from build123d import *
from OCP.BRepFilletAPI import BRepFilletAPI_MakeChamfer

# Parameters (mm, degrees)
SKETCH1_W                = 11.43
SKETCH1_H                = 6.096
BASE_EXTRUDE_DEPTH       = 3.81
CHAMFER1_SIZE            = 2.159
CHAMFER1_SIZE2           = 0.380689951
CHAMFER2_SIZE            = 1.27
CHAMFER2_SIZE2           = 0.111110603
CUT_EXTRUDE1_DEPTH       = 0.254
BOSS_EXTRUDE_THIN1_DEPTH = 0.635
CUT_EXTRUDE2_DEPTH       = 0.254
CUT_EXTRUDE3_DEPTH       = 0.254
LPATTERN1_COUNT          = 4
LPATTERN1_PITCH          = 2.54
MIRROR1_COPY_1_DEPTH     = 0.635
MIRROR1_COPY_2_DEPTH     = 0.635
MIRROR1_COPY_3_DEPTH     = 0.635
MIRROR1_COPY_4_DEPTH     = 0.254
MIRROR1_COPY_5_DEPTH     = 0.254
MIRROR1_COPY_6_DEPTH     = 0.254
MIRROR1_COPY_7_DEPTH     = 0.254
MIRROR1_COPY_8_DEPTH     = 0.254
MIRROR1_COPY_9_DEPTH     = 0.254


with BuildPart() as part:
    # Sketch1 → Base-Extrude (new body)
    with BuildSketch(Plane(origin=(0, 0.381, 0), x_dir=(0, 0, -1), z_dir=(0, 1, 0))):
        with Locations((-3.81, -3.81)):
            Rectangle(SKETCH1_W, SKETCH1_H)
    extrude(amount=BASE_EXTRUDE_DEPTH)

    # Chamfer1: one chamfer whose edges measure the first distance from different faces: ONE call of the kernel's chamfer builder (chamfer() names one face for all edges)
    chamfer1_edges_1 = [part.edges().sort_by_distance(p)[0] for p in [
        (3.81, 4.191, 9.525),
    ]]
    chamfer1_side_1 = [part.faces().sort_by_distance(p)[0] for p in [
        (3.81, 2.286, 9.525),
    ]]
    chamfer1_edges_2 = [part.edges().sort_by_distance(p)[0] for p in [
        (6.858, 4.191, 3.81),
    ]]
    chamfer1_side_2 = [part.faces().sort_by_distance(p)[0] for p in [
        (6.858, 2.286, 3.81),
    ]]
    chamfer1_edges_3 = [part.edges().sort_by_distance(p)[0] for p in [
        (3.81, 4.191, -1.905),
    ]]
    chamfer1_side_3 = [part.faces().sort_by_distance(p)[0] for p in [
        (3.81, 2.286, -1.905),
    ]]
    chamfer1_edges_4 = [part.edges().sort_by_distance(p)[0] for p in [
        (0.762, 4.191, 3.81),
    ]]
    chamfer1_side_4 = [part.faces().sort_by_distance(p)[0] for p in [
        (0.762, 2.286, 3.81),
    ]]
    chamfer1 = BRepFilletAPI_MakeChamfer(part.part.solid().wrapped)
    for e in chamfer1_edges_1:
        chamfer1.Add(CHAMFER1_SIZE, CHAMFER1_SIZE2, e.wrapped, chamfer1_side_1[0].wrapped)  # the first distance lies on this face
    for e in chamfer1_edges_2:
        chamfer1.Add(CHAMFER1_SIZE, CHAMFER1_SIZE2, e.wrapped, chamfer1_side_2[0].wrapped)  # the first distance lies on this face
    for e in chamfer1_edges_3:
        chamfer1.Add(CHAMFER1_SIZE, CHAMFER1_SIZE2, e.wrapped, chamfer1_side_3[0].wrapped)  # the first distance lies on this face
    for e in chamfer1_edges_4:
        chamfer1.Add(CHAMFER1_SIZE, CHAMFER1_SIZE2, e.wrapped, chamfer1_side_4[0].wrapped)  # the first distance lies on this face
    add(Compound.cast(chamfer1.Shape()), mode=Mode.REPLACE)

    # Chamfer2: one chamfer whose edges measure the first distance from different faces: ONE call of the kernel's chamfer builder (chamfer() names one face for all edges)
    chamfer2_edges_1 = [part.edges().sort_by_distance(p)[0] for p in [
        (6.858, 0.381, 3.81),
    ]]
    chamfer2_side_1 = [part.faces().sort_by_distance(p)[0] for p in [
        (6.858, 1.2065, 3.81),
    ]]
    chamfer2_edges_2 = [part.edges().sort_by_distance(p)[0] for p in [
        (3.81, 0.381, 9.525),
    ]]
    chamfer2_side_2 = [part.faces().sort_by_distance(p)[0] for p in [
        (3.81, 1.2065, 9.525),
    ]]
    chamfer2_edges_3 = [part.edges().sort_by_distance(p)[0] for p in [
        (0.762, 0.381, 3.81),
    ]]
    chamfer2_side_3 = [part.faces().sort_by_distance(p)[0] for p in [
        (0.762, 1.2065, 3.81),
    ]]
    chamfer2_edges_4 = [part.edges().sort_by_distance(p)[0] for p in [
        (3.81, 0.381, -1.905),
    ]]
    chamfer2_side_4 = [part.faces().sort_by_distance(p)[0] for p in [
        (3.81, 1.2065, -1.905),
    ]]
    chamfer2 = BRepFilletAPI_MakeChamfer(part.part.solid().wrapped)
    for e in chamfer2_edges_1:
        chamfer2.Add(CHAMFER2_SIZE, CHAMFER2_SIZE2, e.wrapped, chamfer2_side_1[0].wrapped)  # the first distance lies on this face
    for e in chamfer2_edges_2:
        chamfer2.Add(CHAMFER2_SIZE, CHAMFER2_SIZE2, e.wrapped, chamfer2_side_2[0].wrapped)  # the first distance lies on this face
    for e in chamfer2_edges_3:
        chamfer2.Add(CHAMFER2_SIZE, CHAMFER2_SIZE2, e.wrapped, chamfer2_side_3[0].wrapped)  # the first distance lies on this face
    for e in chamfer2_edges_4:
        chamfer2.Add(CHAMFER2_SIZE, CHAMFER2_SIZE2, e.wrapped, chamfer2_side_4[0].wrapped)  # the first distance lies on this face
    add(Compound.cast(chamfer2.Shape()), mode=Mode.REPLACE)

    # Sketch2 → Cut-Extrude1 (cut)
    with BuildSketch(Plane(origin=(0, 4.191, 0), x_dir=(-1, 0, 0), z_dir=(0, 1, 0))):
        with BuildLine():
            Line((-2.794, -2.791910465), (-4.826, -2.791910465))
            Line((-4.826, -2.791910465), (-4.826, -0.508310049))
            ThreePointArc((-4.826, -0.508310049), (-3.81, 0.507689951), (-2.794, -0.508310049))
            Line((-2.794, -0.508310049), (-2.794, -2.791910465))
        make_face()
    extrude(amount=-CUT_EXTRUDE1_DEPTH, mode=Mode.SUBTRACT)

    # Sketch3 → Boss-Extrude-Thin1 (add, symmetric)
    with BuildSketch(Plane(origin=(9.017, 0, 0), x_dir=(-1, 0, 0), z_dir=(0, 0, -1))):
        with BuildLine():
            Line((6.913298214, 1.778), (8.509, 1.778))
            ThreePointArc((8.509, 1.778), (8.778407684, 1.666407684), (8.89, 1.397))
            Line((8.89, 1.397), (8.89, -2.667))
            Line((8.89, -2.667), (9.144, -2.667))
            Line((9.144, -2.667), (9.144, 1.397))
            ThreePointArc((9.144, 1.397), (8.958012806, 1.846012806), (8.509, 2.032))
            Line((8.509, 2.032), (6.913298214, 2.032))
            Line((6.913298214, 2.032), (6.913298214, 1.778))
        make_face()
    boss_extrude_thin1 = extrude(amount=BOSS_EXTRUDE_THIN1_DEPTH, both=True)

    # Sketch4 → Cut-Extrude2 (cut)
    with BuildSketch(Plane(origin=(0.127, 0, 0), x_dir=(0, 0, -1), z_dir=(1, 0, 0))):
        Polygon((-0.635, 0.2794), (-0.2286, 0), (-0.2286, -2.309519874), (0, -2.667), (-0.635, -2.667), align=None)
    cut_extrude2 = extrude(amount=-CUT_EXTRUDE2_DEPTH, mode=Mode.SUBTRACT)

    # Sketch5 → Cut-Extrude3 (cut)
    with BuildSketch(Plane(origin=(0.127, 0, 0), x_dir=(0, 0, -1), z_dir=(1, 0, 0))):
        Polygon((0.635, -2.667), (0, -2.667), (0.2286, -2.309519874), (0.2286, 0), (0.635, 0.2794), align=None)
    cut_extrude3 = extrude(amount=-CUT_EXTRUDE3_DEPTH, mode=Mode.SUBTRACT)

    # LPattern1: Boss-Extrude-Thin1, Cut-Extrude2, Cut-Extrude3 ×4
    with Locations(*[(0, 0, i * LPATTERN1_PITCH) for i in range(1, LPATTERN1_COUNT)]):
        add(boss_extrude_thin1)
        add(cut_extrude2, mode=Mode.SUBTRACT)
        add(cut_extrude3, mode=Mode.SUBTRACT)

    # Mirror1: Boss-Extrude-Thin1, Cut-Extrude2, Cut-Extrude3 across plane
    add(boss_extrude_thin1.mirror(Plane.ZY.offset(-3.81)))
    add(cut_extrude2.mirror(Plane.ZY.offset(-3.81)), mode=Mode.SUBTRACT)
    add(cut_extrude3.mirror(Plane.ZY.offset(-3.81)), mode=Mode.SUBTRACT)

    # Mirror1 copy 1 sketch → Mirror1 copy 1 (add, symmetric)
    with BuildSketch(Plane(origin=(-1.397, 0, 2.54), x_dir=(1, 0, 0), z_dir=(0, 0, -1))):
        with BuildLine():
            Line((6.913298214, -1.778), (8.509, -1.778))
            ThreePointArc((8.509, -1.778), (8.778407684, -1.666407684), (8.89, -1.397))
            Line((8.89, -1.397), (8.89, 2.667))
            Line((8.89, 2.667), (9.144, 2.667))
            Line((9.144, 2.667), (9.144, -1.397))
            ThreePointArc((9.144, -1.397), (8.958012806, -1.846012806), (8.509, -2.032))
            Line((8.509, -2.032), (6.913298214, -2.032))
            Line((6.913298214, -2.032), (6.913298214, -1.778))
        make_face()
    extrude(amount=MIRROR1_COPY_1_DEPTH, both=True)

    # Mirror1 copy 2 sketch → Mirror1 copy 2 (add, symmetric)
    with BuildSketch(Plane(origin=(-1.397, 0, 5.08), x_dir=(1, 0, 0), z_dir=(0, 0, -1))):
        with BuildLine():
            Line((6.913298214, -1.778), (8.509, -1.778))
            ThreePointArc((8.509, -1.778), (8.778407684, -1.666407684), (8.89, -1.397))
            Line((8.89, -1.397), (8.89, 2.667))
            Line((8.89, 2.667), (9.144, 2.667))
            Line((9.144, 2.667), (9.144, -1.397))
            ThreePointArc((9.144, -1.397), (8.958012806, -1.846012806), (8.509, -2.032))
            Line((8.509, -2.032), (6.913298214, -2.032))
            Line((6.913298214, -2.032), (6.913298214, -1.778))
        make_face()
    extrude(amount=MIRROR1_COPY_2_DEPTH, both=True)

    # Mirror1 copy 3 sketch → Mirror1 copy 3 (add, symmetric)
    with BuildSketch(Plane(origin=(-1.397, 0, 7.62), x_dir=(1, 0, 0), z_dir=(0, 0, -1))):
        with BuildLine():
            Line((6.913298214, -1.778), (8.509, -1.778))
            ThreePointArc((8.509, -1.778), (8.778407684, -1.666407684), (8.89, -1.397))
            Line((8.89, -1.397), (8.89, 2.667))
            Line((8.89, 2.667), (9.144, 2.667))
            Line((9.144, 2.667), (9.144, -1.397))
            ThreePointArc((9.144, -1.397), (8.958012806, -1.846012806), (8.509, -2.032))
            Line((8.509, -2.032), (6.913298214, -2.032))
            Line((6.913298214, -2.032), (6.913298214, -1.778))
        make_face()
    extrude(amount=MIRROR1_COPY_3_DEPTH, both=True)

    # Mirror1 copy 4 sketch → Mirror1 copy 4 (cut)
    with BuildSketch(Plane(origin=(7.493, 0, 2.54), x_dir=(0, 0, -1), z_dir=(-1, 0, 0))):
        Polygon((-0.635, -0.2794), (-0.2286, 0), (-0.2286, 2.309519874), (0, 2.667), (-0.635, 2.667), align=None)
    extrude(amount=-MIRROR1_COPY_4_DEPTH, mode=Mode.SUBTRACT)

    # Mirror1 copy 5 sketch → Mirror1 copy 5 (cut)
    with BuildSketch(Plane(origin=(7.493, 0, 5.08), x_dir=(0, 0, -1), z_dir=(-1, 0, 0))):
        Polygon((-0.635, -0.2794), (-0.2286, 0), (-0.2286, 2.309519874), (0, 2.667), (-0.635, 2.667), align=None)
    extrude(amount=-MIRROR1_COPY_5_DEPTH, mode=Mode.SUBTRACT)

    # Mirror1 copy 6 sketch → Mirror1 copy 6 (cut)
    with BuildSketch(Plane(origin=(7.493, 0, 7.62), x_dir=(0, 0, -1), z_dir=(-1, 0, 0))):
        Polygon((-0.635, -0.2794), (-0.2286, 0), (-0.2286, 2.309519874), (0, 2.667), (-0.635, 2.667), align=None)
    extrude(amount=-MIRROR1_COPY_6_DEPTH, mode=Mode.SUBTRACT)

    # Mirror1 copy 7 sketch → Mirror1 copy 7 (cut)
    with BuildSketch(Plane(origin=(7.493, 0, 2.54), x_dir=(0, 0, -1), z_dir=(-1, 0, 0))):
        Polygon((0.635, 2.667), (0, 2.667), (0.2286, 2.309519874), (0.2286, 0), (0.635, -0.2794), align=None)
    extrude(amount=-MIRROR1_COPY_7_DEPTH, mode=Mode.SUBTRACT)

    # Mirror1 copy 8 sketch → Mirror1 copy 8 (cut)
    with BuildSketch(Plane(origin=(7.493, 0, 5.08), x_dir=(0, 0, -1), z_dir=(-1, 0, 0))):
        Polygon((0.635, 2.667), (0, 2.667), (0.2286, 2.309519874), (0.2286, 0), (0.635, -0.2794), align=None)
    extrude(amount=-MIRROR1_COPY_8_DEPTH, mode=Mode.SUBTRACT)

    # Mirror1 copy 9 sketch → Mirror1 copy 9 (cut)
    with BuildSketch(Plane(origin=(7.493, 0, 7.62), x_dir=(0, 0, -1), z_dir=(-1, 0, 0))):
        Polygon((0.635, 2.667), (0, 2.667), (0.2286, 2.309519874), (0.2286, 0), (0.635, -0.2794), align=None)
    extrude(amount=-MIRROR1_COPY_9_DEPTH, mode=Mode.SUBTRACT)


solid = part.part
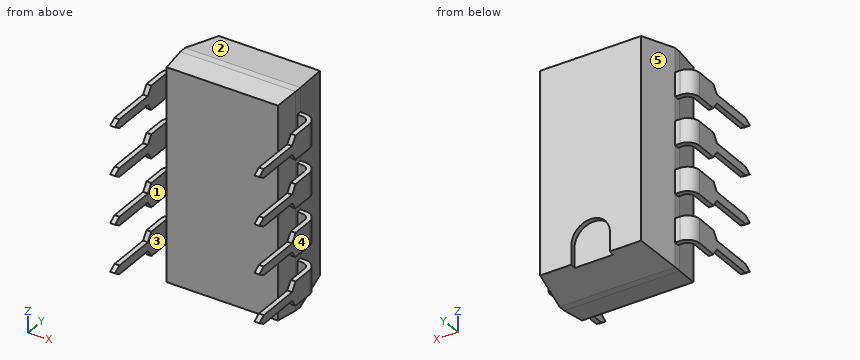
CAD build for the part. Positions are in the model's coordinates, mm. Face numbers are marked on the shaded views. A direction names the side the tool comes from. Coordinates: 2 decimals unless noted, no trailing zeros. Write each loop counter-clockwise with the first axis right and the second up, starting at its lowest first coordinate (ties: lowest second). Pieces come first, ordered by that corner, then holes. Notation, with made-up numbers: M 18,80.5 L 59,80.5 A24 cw 59,93.5 Z; hole C 26,-18 d2. An arc over 180 degrees is marked long. Return JSON: item names as keys, results as strings.
Item 1: Probe line 1 (X direction, y = 2, z = -1); line 2 (Y direction, x = 5, z = 2.5); line 3 (X direction, y = 3.25, z = 4). List the from-to ranges inside material, lowest first. Write a range as from..to.
Findings below:
{"line 1": "x = 0.76..6.86", "line 2": "y = 0.38..4.19", "line 3": "x = 0.98..6.64"}
Item 2: Drop a flat-ended pin along its axis: pin 1 Ø0.7 at (x, y) = (0.5, 1) entering from +Z. Give the stop position or say it passes through.
Findings below:
{"pin 1": "stops at z = 9.48"}
Item 3: Which spindle directions (+Z, -Z, +X, -X, +Y, -Y) get a long thin tool onto all of the face, cutting with end or side? Do the marked faces 1 and 2. Say none if no direction does.
Findings below:
{"face 1": "+Z, -Z, -Y", "face 2": "+Z, +X, -X, +Y"}
Item 4: Two-plate mould, pull along X, no slides. Class the marked faces 3, 4 and 5: +X half, -X half, draft (parallel to the pull), parting line (faces both ways), or undercut.
Findings below:
{"face 3": "undercut", "face 4": "+X half", "face 5": "-X half"}
Item 5: Slice it at D-D, the plane z = 7.25. Write the cut outline in (x, y) (3 decimals), and give its area (3 significant figures).
Findings below:
{"outline": "M -0.127,0.097 L 0.127,0.097 L 0.127,1.397 A0.381 cw 0.508,1.778 L 0.762,1.778 L 0.762,1.651 L 0.873,0.381 L 6.747,0.381 L 6.858,1.651 L 6.858,1.778 L 7.112,1.778 A0.381 cw 7.493,1.397 L 7.493,0.097 L 7.747,0.097 L 7.747,1.397 A0.635 ccw 7.112,2.032 L 6.858,2.032 L 6.477,4.191 L 1.143,4.191 L 0.762,2.032 L 0.508,2.032 A0.635 ccw -0.127,1.397 Z", "area": "23.5 mm2"}
Item 6: Slice it at B-B, the plane x = 5.5. Write the cut outline in (y, z) (3 decimals), and give its area (3 significant figures).
Findings below:
{"outline": "M 0.381,-1.794 L 1.651,-1.905 L 2.032,-1.905 L 4.191,-1.524 L 4.191,9.144 L 2.032,9.525 L 1.651,9.525 L 0.381,9.414 Z", "area": "42.6 mm2"}
Item 7: Slice it at A-A, the plane y = -0.5. State how many separate pieces and enclosed holes the cut face has, and give its area (3 significant figures).
Findings below:
{"separate pieces": "8", "enclosed holes": "0", "area": "0.929 mm2"}
Item 8: Slice it at C-C, the plane x = 7.25. Write the cut outline in (y, z) (3 decimals), and give its area (3 significant figures).
Findings below:
{"outline": "M 1.752,-0.635 L 2.017,-0.635 L 2.017,0.635 L 1.752,0.635 Z; M 1.752,1.905 L 2.017,1.905 L 2.017,3.175 L 1.752,3.175 Z; M 1.752,4.445 L 2.017,4.445 L 2.017,5.715 L 1.752,5.715 Z; M 1.752,6.985 L 2.017,6.985 L 2.017,8.255 L 1.752,8.255 Z", "area": "1.34 mm2"}
